```python
from build123d import *

# Parameters (mm, degrees)
SKETCH1_W           = 50.8
SKETCH1_H           = 50.8
BOSS_EXTRUDE1_DEPTH = 50.8
SHELL1_T            = -3
SKETCH2_R           = 3.175
CUT_EXTRUDE1_DEPTH  = 50.8
SKETCH3_R           = 12.5
CUT_EXTRUDE2_DEPTH  = 49.8
SKETCH4_W           = 25
SKETCH4_H           = 6
CUT_EXTRUDE3_DEPTH  = 49.8


with BuildPart() as part:
    # Sketch1 → Boss-Extrude1 (new body)
    with BuildSketch(Plane(origin=(0, 0, 0), x_dir=(1, 0, 0), z_dir=(0, 1, 0))):
        Rectangle(SKETCH1_W, SKETCH1_H)
    extrude(amount=BOSS_EXTRUDE1_DEPTH)

    # Shell1
    shell1_openings = [part.faces().sort_by_distance(p)[0] for p in [
        (25.4, 25.4, 0),
    ]]
    offset(amount=SHELL1_T, openings=shell1_openings, kind=Kind.INTERSECTION)

    # Sketch2 → Cut-Extrude1 (cut)
    with BuildSketch(Plane.ZY.offset(25.4)):
        with Locations((0, 25.4)):
            Circle(SKETCH2_R)
    extrude(amount=-CUT_EXTRUDE1_DEPTH, mode=Mode.SUBTRACT)

    # Sketch3 → Cut-Extrude2 (cut)
    with BuildSketch(Plane(origin=(0, 50.8, 0), x_dir=(1, 0, 0), z_dir=(0, 1, 0))):
        with Locations(Location((0, 0, 0), (0, 0, 270))):
            Circle(SKETCH3_R)
    extrude(amount=-CUT_EXTRUDE2_DEPTH, mode=Mode.SUBTRACT)

    # Sketch4 → Cut-Extrude3 (cut)
    with BuildSketch(Plane(origin=(-22.4, 0, 0), x_dir=(0, 0, -1), z_dir=(1, 0, 0))):
        with Locations((0, 43.442725036)):
            Rectangle(SKETCH4_W, SKETCH4_H)
    extrude(amount=-CUT_EXTRUDE3_DEPTH, mode=Mode.SUBTRACT)


solid = part.part
```
Geometry: final body of the model. Coordinates: model frame, mm. A direction names the side the tool comes from. Coordinates: 2 decimals unless noted, no trailing zeros. Order: outer loops, then holes, each group sorted by start corner. A loop starts at its lowest first (then second) coordinate and runs counter-clockwise, first axis right, second up.
Item 1: Section query A-A (x = -20.5). Output: boundary loops of the cut face in (y, z).
Answer:
outline: (0, -25.4) - (50.8, -25.4) - (50.8, 25.4) - (0, 25.4) - close; hole (3, -22.4) - (47.8, -22.4) - (47.8, 22.4) - (3, 22.4) - close
Item 2: Material intervals for line 1 along Y through (x, z) = (-24, 0) (3 decimals); line 2 along Y through (x, z) = (15, -1.5); line 3 along Z through (x, y) = (-8, 25), sorted ascending.
Answer:
line 1: y = 0 to 22.225, 28.575 to 40.443, 46.443 to 50.8
line 2: y = 0 to 3, 47.8 to 50.8
line 3: z = -25.4 to -22.4, 22.4 to 25.4
Item 3: Section query B-B (y = 25.4). Output: boundary loops of the cut face in (x, z) (3 decimals).
Answer:
outline: (-25.4, -25.4) - (25.4, -25.4) - (25.4, -22.4) - (-22.4, -22.4) - (-22.4, -3.175) - (-25.4, -3.175) - close; (-25.4, 3.175) - (-22.4, 3.175) - (-22.4, 22.4) - (25.4, 22.4) - (25.4, 25.4) - (-25.4, 25.4) - close
Item 4: Section query C-C (z = 0). Output: boundary loops of the cut face in (x, y) (3 decimals).
Answer:
outline: (-25.4, 0) - (25.4, 0) - (25.4, 3) - (12.5, 3) - (12.5, 1) - (-12.5, 1) - (-12.5, 3) - (-22.4, 3) - (-22.4, 22.225) - (-25.4, 22.225) - close; (-25.4, 28.575) - (-22.4, 28.575) - (-22.4, 40.443) - (-25.4, 40.443) - close; (-25.4, 46.443) - (-22.4, 46.443) - (-22.4, 47.8) - (-12.5, 47.8) - (-12.5, 50.8) - (-25.4, 50.8) - close; (12.5, 47.8) - (25.4, 47.8) - (25.4, 50.8) - (12.5, 50.8) - close
Item 5: Contact query for a flat-ended pin moving along its axis: P1, Ø1.5, axis at y = 22.5, z = 14, coming from the +X side. Output: stop coordinate, or through.
Answer:
P1: stops at x = -22.4
Item 6: Section query D-D (z = 14.5). Output: boundary loops of the cut face in (x, y).
Answer:
outline: (-25.4, 0) - (25.4, 0) - (25.4, 3) - (-22.4, 3) - (-22.4, 47.8) - (25.4, 47.8) - (25.4, 50.8) - (-25.4, 50.8) - close
Item 7: Access query for faces 1 (the face through (25.4, 25, 23)), 2 (the face through (-24, 40.443, 0)), 3 (the face through (1, 25, 22.4)), 4 (the face through (0, 1, 0)). Directions: +Z, -Z, +X, -X, +Y, -Y. A direction counts if a zero-diameter tool reaches every point of the face in a straight line with its end or side. Return the directions, or none.
Answer:
face 1: +Z, -Z, +X, +Y, -Y
face 2: +X, -X
face 3: +X
face 4: +Y
Item 8: Draft query along X for faces 5 (the face through (-22.4, 20, 0)), 6 (the face through (-25.4, 19, 0)), 7 (the face through (12, 3, -5)), 8 (the face through (3.755, 49.321, 11.923)). Return one class per face: released by +X, released by -X, zero draft, split by the parting line, or undercut.
Answer:
face 5: released by +X
face 6: released by -X
face 7: zero draft
face 8: undercut
